Could you check a few things on this model? Use its own coordinates, in mm. A direction names the side the tool comes from. Give positions to 0.01 mm unless a question says otherwise; leave off trailing zeros. Write each loop counter-clockwise with the first axis right and the second up, starting at its lowest first coordinate (ties: lowest second). Pieces come first, ordered by that corner, then holes. Notation, with made-up numbers: M -15.5,-0.5 L 9.5,-0.5 A16 cw 9.5,9.5 Z; hole C 29.25,38 d2. An arc over 180 degrees is marked long. Use one line per item in the form item = value.
from build123d import *

# Parameters (mm, degrees)
F0_W           = 76.2
F0_H           = 50.8
F1_DEPTH       = 8.255
F2_R           = 2.402553
F3_DEPTH       = 9.525
F5_D           = 5.1054
F5_CSINK_D     = 7.62
F5_CSINK_ANGLE = 82


with BuildPart() as f1:
    # F0 (on Right) → F1 (new body)
    with BuildSketch(Plane.YZ):
        Rectangle(F0_W, F0_H)
    extrude(amount=F1_DEPTH)

    # F2 (on face) → F3 (cut)
    with BuildSketch(Plane.XZ.offset(38.1)):
        with Locations((3.510773, 9.267487)):
            Circle(F2_R)
    extrude(amount=-F3_DEPTH, mode=Mode.SUBTRACT)

    # F5 (through all)
    with Locations(Plane.YZ.offset(8.255)):
        with Locations((28.575, 15.875)):
            CounterSinkHole(F5_D / 2, F5_CSINK_D / 2, counter_sink_angle=F5_CSINK_ANGLE)


solid = f1.part
1) If I drill on L1, parallel to Z at x = 3.5, y = 29; L2, parallel to Y at x = 2.75, z = 18; L3, parallel to Y at x = 2.5, z = 17.5, over which ranges is the centre line in solid material (lowest first)?
Checked values:
L1 = -25.4 to 13.36, 18.39 to 25.4
L2 = -38.1 to 27.16, 29.99 to 38.1
L3 = -38.1 to 26.61, 30.54 to 38.1
2) I want a section at B-B, the plane z = 8.5. Please give me the cut outline in (x, y) (3 decimals), plus the area to 3 significant figures.
Checked values:
outline = M 0,-38.1 L 1.234,-38.1 L 1.234,-28.575 L 5.787,-28.575 L 5.787,-38.1 L 8.255,-38.1 L 8.255,38.1 L 0,38.1 Z
area = 586 mm2
3) For faces 4 (the cylindrical face through (3.2, -33.4, 11.65)), 5 (the cylindrical face through (3.357, 27.203, 18.027)), which set-ups out of +Z, -Z, +X, -X, +Y, -Y let a thin tool reach every point of the face, with its end or its side?
Checked values:
face_4 = -Y
face_5 = +X, -X
4) I want a section at C-C, the plane y = -32. Please give me the cut outline in (x, z) (3 decimals).
Checked values:
outline = M 0,-25.4 L 8.255,-25.4 L 8.255,25.4 L 0,25.4 Z; hole C 3.511,9.267 d4.805
5) I want a section at A-A, the plane x = 4.75. Please give me the cut outline in (y, z) (3 decimals), plus the area to 3 significant figures.
Checked values:
outline = M -38.1,-25.4 L 38.1,-25.4 L 38.1,25.4 L -38.1,25.4 L -38.1,11.326 L -28.575,11.326 L -28.575,7.209 L -38.1,7.209 Z; hole C 28.575,15.875 d5.105
area = 3,810 mm2
6) For pin 1 Ø4 at (y, z) = (28.575, 15.875) entering from +X, with a flat end and sliding along its axis, tell me the tip position at first contact or that it passes through.
Checked values:
pin_1 = through
7) Thinking about a two-plate mould opening in Z: for faces 1 (the flat face through (4, -1, -25.4)), 2 (the flat face through (3, -28.575, 9)), 3 (the flat face through (4, 38.1, 0)), which applies, released by +Z, released by -Z, zero draft, split by the parting line, or undercut?
Checked values:
face_1 = released by -Z
face_2 = undercut
face_3 = zero draft
